The listing builds one solid part. Answer for the finished solid, in the listing's coordinates (mm). Face numbers are marked on the shaded views. A direction names the side the tool comes from. Coordinates: 2 decimals unless noted, no trailing zeros. Order: outer loops, then holes, each group sorted by start corner. A loop starts at its lowest first (then second) coordinate and runs counter-clockwise, first axis right, second up. Notation, with made-up numbers: M 30.25,60.5 L 46.25,60.5 A16 ccw 46.25,89.5 Z; hole C -14.5,-24.75 d8. An arc over 180 degrees is marked long. One line per item, written item: value. Start each with the question number.
Q1. The part is cut by section C-C on y = 14. Give the vertices of the cut face in (x, z).
Q2. The part is cut by section D-D on z = 7.5. Give the vertices of the cut face in (x, y), then the cut area to 3 significant figures.
Q3. Straight lines are drawn through the part: line 1 along X through (y, z) = (-2.05, 15); line 2 along X through (y, z) = (1, 17.5); line 3 along Y through (x, z) = (6, 22.5). For each, find the intervals that lie inside material, in ascending order. Write a range as [from, to].
Q4. Each of these flat-tipped pins is pushed along its axis until it touches: pin 1 Ø5 at (x, y) = (14.5, 9) entering from -Z; pin 2 Ø4 at (x, z) = (22.5, 15) entering from +Y; pin 3 Ø12 at (x, y) = (-16.5, 9) entering from -Z; pin 4 Ø3 at (y, z) = (2.5, 21.5) entering from +X. Where does it stop, or does it pass through?
Q5. The part is cut by section A-A on z = 16.25. Give the vertices of the cut face in (x, y).
Q6. For the marked faces 1, 2 and 3, determine the directions among +Z, -Z, +X, -X, +Y, -Y from which every point of the face is accessible in a straight line to the end or side of a thin tool.
Q7. Determine the mould class of the marked faces 4, 5 and 6 for opening direction X: pulls with the +X half, pulls with the -X half, needs draft (parallel to the pull), parting line crosses it, or undercut.
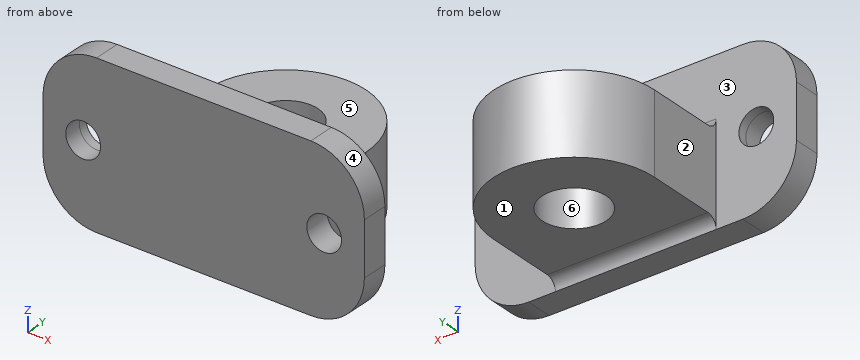
```python
from build123d import *

# Parameters (mm, degrees)
SKETCH_1_R          = 6
EXTRUDE_1_DEPTH     = 30
SKETCH_2_W          = 13
SKETCH_2_H          = 30
SKETCH_2_W_2        = 2
CUT_EXTRUDE_1_DEPTH = 15
SKETCH_3_R          = 3.25
CUT_EXTRUDE_2_DEPTH = 15
FILLET_1_R          = 2
FILLET_2_R          = 10


with BuildPart() as part:
    # 草图1 → 凸台-拉伸1 (new body)
    with BuildSketch(Plane.XY):
        with BuildLine():
            Line((-30, 1.666666667), (-15, 1.666666667))
            Line((-15, 1.666666667), (-15, 16.666666667))
            ThreePointArc((-15, 16.666666667), (0, 31.666666667), (15, 16.666666667))
            Line((15, 16.666666667), (15, 1.666666667))
            Line((15, 1.666666667), (30, 1.666666667))
            Line((30, 1.666666667), (30, -3.333333333))
            Line((30, -3.333333333), (-30, -3.333333333))
            Line((-30, -3.333333333), (-30, 1.666666667))
        make_face()
        with Locations((0, 16.666666667)):
            Circle(SKETCH_1_R, mode=Mode.SUBTRACT)
    extrude(amount=EXTRUDE_1_DEPTH)

    # 草图2 → 切除-拉伸1 (cut, symmetric)
    with BuildSketch(Plane(origin=(0, 0, 0), x_dir=(0, 0, -1), z_dir=(1, 0, 0))):
        with Locations((-23.5, 16.666666667)):
            Rectangle(SKETCH_2_W, SKETCH_2_H)
        with Locations((-1, 16.666666667)):
            Rectangle(SKETCH_2_W_2, SKETCH_2_H)
    extrude(amount=CUT_EXTRUDE_1_DEPTH, both=True, mode=Mode.SUBTRACT)

    # 草图3 → 切除-拉伸2 (cut, symmetric)
    with BuildSketch(Plane(origin=(0, 0, 0), x_dir=(1, 0, 0), z_dir=(0, 1, 0))):
        with Locations((-22.5, -15)):
            Circle(SKETCH_3_R)
        with Locations((22.5, -15)):
            Circle(SKETCH_3_R)
    extrude(amount=CUT_EXTRUDE_2_DEPTH, both=True, mode=Mode.SUBTRACT)

    # 圆角1
    fillet_1_edges = [part.edges().sort_by_distance(p)[0] for p in [
        (0, 1.666666667, 17),
        (0, 1.666666667, 2),
    ]]
    fillet(fillet_1_edges, radius=FILLET_1_R - 0.0001)  # a hair under: the kernel refuses the full size

    # 圆角2
    fillet_2_edges = [part.edges().sort_by_distance(p)[0] for p in [
        (30, -0.833333333, 30),
        (-30, -0.833333333, 0),
        (-30, -0.833333333, 30),
        (30, -0.833333333, 0),
    ]]
    fillet(fillet_2_edges, radius=FILLET_2_R)


solid = part.part
```
Output:
1. outline: M -15,2 L -5.37,2 L -5.37,17 L -15,17 Z; M 5.37,2 L 15,2 L 15,17 L 5.37,17 Z
2. outline: M -29.68,-3.33 L 29.68,-3.33 L 29.68,1.67 L 15,1.67 L 15,16.67 A15 ccw -15,16.67 L -15,1.67 L -29.68,1.67 Z; hole C 0,16.67 d12
2. area: 987 mm^2
3. line 1: x = [-30, -25.75], [-19.25, 19.25], [25.75, 30]
3. line 2: x = [-30, -24.58], [-20.42, 20.42], [24.58, 30]
3. line 3: y = [-3.33, 1.67]
4. pin 1: stops at z = 2
4. pin 2: passes through
4. pin 3: stops at z = 1.94
4. pin 4: stops at x = 30
5. outline: M -30,-3.33 L -25.5,-3.33 L -25.5,1.67 L -30,1.67 Z; M -19.5,-3.33 L 19.5,-3.33 L 19.5,1.67 L 15,1.67 L 15,16.67 A15 ccw -15,16.67 L -15,1.67 L -19.5,1.67 Z; M 25.5,-3.33 L 30,-3.33 L 30,1.67 L 25.5,1.67 Z; hole C 0,16.67 d12
6. face 1: -Z, +X, -X, +Y
6. face 2: +Z, -Z, -X, +Y
6. face 3: +Z, +Y
7. face 4: pulls with the +X half
7. face 5: needs draft
7. face 6: undercut
